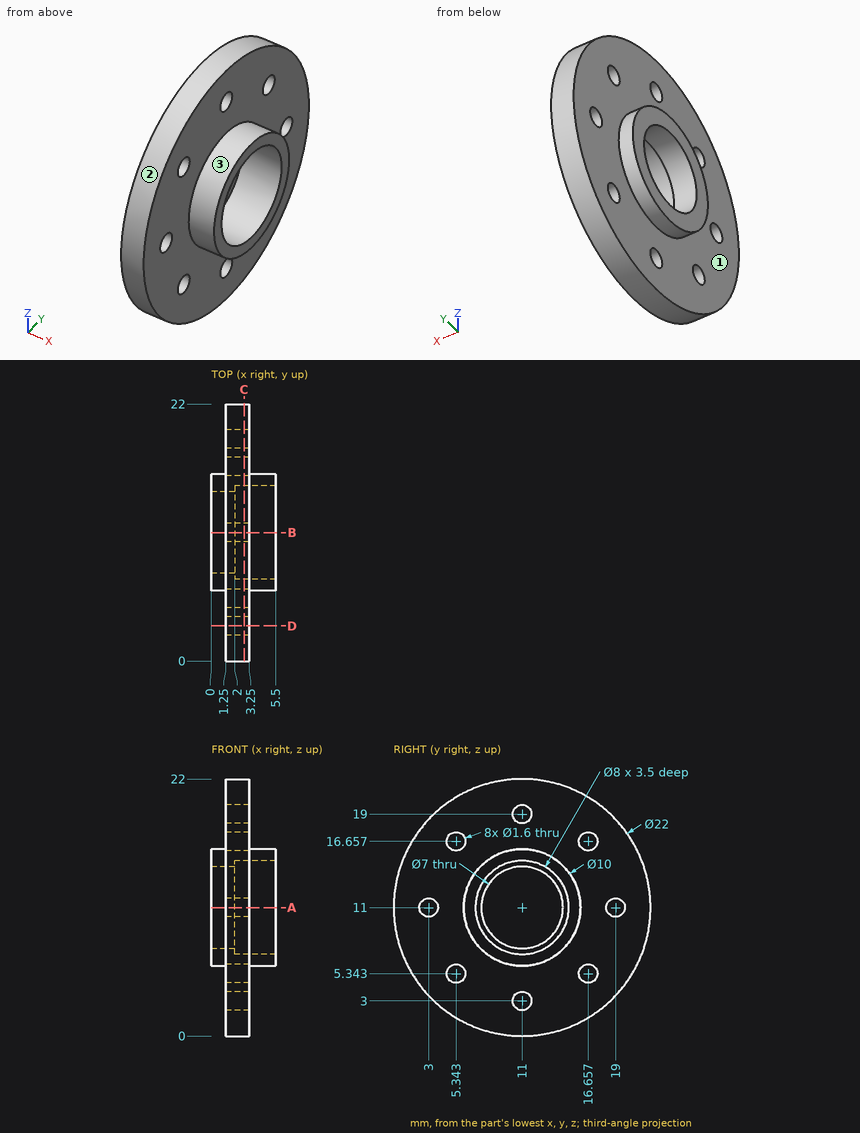
Could you check a few things on this drawing? It's one solid part, dimensions in mm from its lowest x, y, z. A direction names the side the tool comes from. Round coordinates to 2 decimals unless told otherwise and drop trailing zeros. Order: outer loops, then holes, each group sorted by start corner. A loop starts at its lowest first (then second) coordinate and runs counter-clockwise, first axis right, second up. Notation, with made-up numbers: M -18,-2.5 L 14,-2.5 A24 ccw 14,13.5 Z; hole C 12.5,80 d5. An arc over 180 degrees is marked long. Return JSON: item names as keys, results as strings. Group by question number.
1. If we section it at C-C on x = 2.8: State how many separate pieces and enclosed holes the cut face has, then the cut area to 3 significant figures.
2. I'm going to push flat-ended pins straight in: pin 1 Ø1.8 at (y, z) = (16.66, 5.34) entering from +X; pin 2 Ø1.8 at (y, z) = (16.66, 16.66) entering from -X; pin 3 Ø3 at (x, z) = (1, 14.5) entering from +Y; pin 4 Ø5 at (y, z) = (11, 11) entering from +X. Where does each tip first touch, or does it pass through?
3. If we section it at D-D on y = 3: List the corners of the cut face in (x, z) for me, then the cut area to 3 significant figures.
4. On a 3-axis mill with a long thin cutter (end or side, diameter ignored), from which of +Z, -Z, +X, -X, +Y, -Y can I reach the whole of each face in a straight line? I mean the marked faces 1, 2 and 3. Say none if no direction works.
5. Please list where these lines run through material, in increasing order: probe 1 along Y at (x, z) = (1.95, 11); probe 2 along Y at (x, z) = (1.3, 5); probe 3 along X at (y, z) = (14.75, 2.75).
6. If we section it at A-A on z = 11: List the corners of the cut face in (x, y) for me.
Reply:
{
 "1": {"separate pieces": "1", "enclosed holes": "9", "area": "314 mm^2"},
 "2": {"pin 1": "x = 3.25", "pin 2": "x = 1.25", "pin 3": "y = 21.81", "pin 4": "through"},
 "3": {"outline": "M 1.25,3.45 L 3.25,3.45 L 3.25,10.2 L 1.25,10.2 Z; M 1.25,11.8 L 3.25,11.8 L 3.25,18.55 L 1.25,18.55 Z", "area": "27.0 mm^2"},
 "4": {"face 1": "-X", "face 2": "+X, -X", "face 3": "+X"},
 "5": {"probe 1": "0 to 2.2, 3.8 to 7.5, 14.5 to 18.2, 19.8 to 22", "probe 2": "1.78 to 4.62, 6.07 to 15.93, 17.38 to 20.22", "probe 3": "1.25 to 3.25"},
 "6": {"outline": "M 0,6 L 1.25,6 L 1.25,3.8 L 3.25,3.8 L 3.25,6 L 5.5,6 L 5.5,7 L 2,7 L 2,7.5 L 0,7.5 Z; M 0,14.5 L 2,14.5 L 2,15 L 5.5,15 L 5.5,16 L 3.25,16 L 3.25,18.2 L 1.25,18.2 L 1.25,16 L 0,16 Z; M 1.25,0 L 3.25,0 L 3.25,2.2 L 1.25,2.2 Z; M 1.25,19.8 L 3.25,19.8 L 3.25,22 L 1.25,22 Z"}
}
